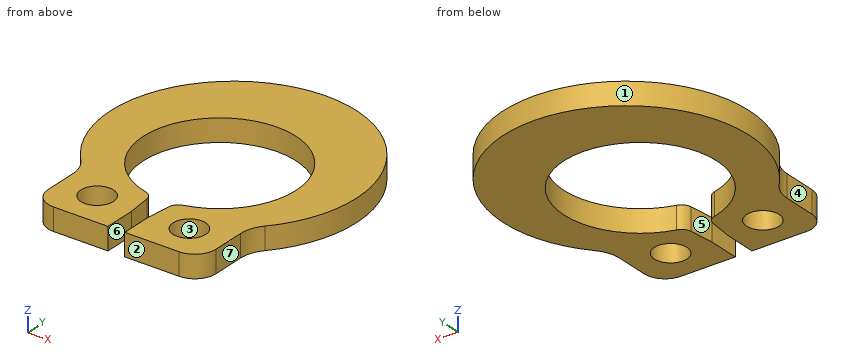
from build123d import *

# Parameters (mm, degrees)
SKETCH3_R               = 0.6477
BOSS_EXTRUDE1_DEPTH     = 0.4445
CUT_EXTRUDE1_DEPTH      = 1.4445
CUT_EXTRUDE1_DEPTH_BACK = 1.4445
FILLET1_R               = 0.4162425


with BuildPart() as part:
    # Sketch3 → Boss-Extrude1 (new body, symmetric)
    with BuildSketch(Plane.XY):
        with BuildLine():
            Line((3.32486, -4.653915), (3.32486, -3.346426518))
            ThreePointArc((3.32486, -3.346426518), (3.408862886, -2.887538523), (3.649976862, -2.488165606))
            ThreePointArc((3.649976862, -2.488165606), (0, 5.6134), (-3.649976862, -2.488165606))
            ThreePointArc((-3.649976862, -2.488165606), (-3.408862886, -2.887538523), (-3.32486, -3.346426518))
            Line((-3.32486, -3.346426518), (-3.32486, -4.653915))
            ThreePointArc((-3.32486, -4.653915), (-3.081030789, -5.242570789), (-2.492375, -5.4864))
            Line((-2.492375, -5.4864), (-0.332486, -5.4864))
            Line((-0.332486, -5.4864), (-0.332486, -3.004257615))
            ThreePointArc((-0.332486, -3.004257615), (0, 3.0226), (0.332486, -3.004257615))
            Line((0.332486, -3.004257615), (0.332486, -5.4864))
            Line((0.332486, -5.4864), (2.492375, -5.4864))
            ThreePointArc((2.492375, -5.4864), (3.081030789, -5.242570789), (3.32486, -4.653915))
        make_face()
        with Locations((-1.828673, -4.057999533)):
            Circle(SKETCH3_R, mode=Mode.SUBTRACT)
        with Locations((1.828673, -4.057999533)):
            Circle(SKETCH3_R, mode=Mode.SUBTRACT)
    extrude(amount=BOSS_EXTRUDE1_DEPTH, both=True)

    # Sketch4 → Cut-Extrude1 (cut, two sides)
    with BuildSketch(Plane.XY) as cut_extrude1_sk:
        Polygon((-0.332486, -4.245328808), (-0.797425121, 0), (0.797425121, 0), (0.332486, -4.245328808), align=None)
    extrude(amount=CUT_EXTRUDE1_DEPTH, mode=Mode.SUBTRACT)
    extrude(cut_extrude1_sk.sketch, amount=-CUT_EXTRUDE1_DEPTH_BACK, mode=Mode.SUBTRACT)

    # Fillet1
    fillet1_edges = [part.edges().sort_by_distance(p)[0] for p in [
        (-0.470430427, -2.985767234, 0),
        (0.470430427, -2.985767234, 0),
    ]]
    fillet(fillet1_edges, radius=FILLET1_R)


solid = part.part
For this review, take the finished solid that the model builds, in its own axes (mm). Face numbers are marked on the shaded views. A direction names the side the tool comes from. Give positions to 0.01 mm unless a question says otherwise; leave off trailing zeros. Loops run counter-clockwise (first coordinate to the right, second up) from the corner with the lowest first, then second, coordinate; pieces in that order, holes last. Notation, with made-up numbers: M 73.25,-25.75 L 130.25,-25.75 A19 cw 130.25,4.25 Z; hole C -30,-39 d6. An arc over 180 degrees is marked long. Put each result on its own line as item: value. Start each with the question number.
(1) For pin 1 (1.7 mm diameter, centred on x = 1.83, y = -4.06, fed in from +Z), flat-tipped, find the tip position at first contact; note if it passes through.
(2) The part is to be moulded in two halves that separate along Y. For the marked faces 1, 2 and 3, say which applies: +Y half, -Y half, draft (parallel to the pull), parting line (faces both ways), or undercut.
(3) Machinability: for the marked faces 4, 5, 6 and 7, which of the approach directions +Z, -Z, +X, -X, +Y, -Y give a long, thin tool a straight path to every point of the face, cutting with its end or side? Answer none if there is none.
(4) Wall thickness on L1, parallel to Y at x = 1.5, z = -0.15; L2, parallel to Y at x = 2, z = -0.4; L3, parallel to X at y = -4, z = 0.15: over which ranges is each line inside the solid? List them lowest first.
(5) Add section C-C, the plane z = 0. Write out the cut boundary in (x, y), then the cut area to 3 significant figures.
(6) Add section B-B, the plane y = 0. Write out the cut boundary in (x, z), then the cut area to 3 significant figures.
(7) Add section D-D, the plane x = 1.5. Write out the cut boundary in (y, z), then the cut area to 3 significant figures.
(8) Add section A-A, the plane x = -2.75. Write out the cut boundary in (y, z).
Result:
1. pin 1: stops at z = 0.44
2. face 1: parting line
2. face 2: -Y half
2. face 3: undercut
3. face 4: +Z, -Z, -X, -Y
3. face 5: +Z, -Z
3. face 6: +Z, -Z, -Y
3. face 7: +Z, -Z, +X, -Y
4. L1: y = -5.49 to -4.62, -3.5 to -2.62, 2.62 to 5.38
4. L2: y = -5.49 to -4.68, -3.43 to -2.27, 2.27 to 5.18
4. L3: x = -3.32 to -2.47, -1.18 to -0.36, 0.36 to 1.18, 2.47 to 3.32
5. outline: M -3.65,-2.49 A1.3 cw -3.32,-3.35 L -3.32,-4.65 A0.83 ccw -2.49,-5.49 L -0.33,-5.49 L -0.33,-4.25 L -0.44,-3.29 A0.42 ccw -0.75,-2.93 A3.02 cw long 0.75,-2.93 A0.42 ccw 0.44,-3.29 L 0.33,-4.25 L 0.33,-5.49 L 2.49,-5.49 A0.83 ccw 3.32,-4.65 L 3.32,-3.35 A1.3 cw 3.65,-2.49 A4.87 ccw long Z; hole C -1.83,-4.06 d1.3; hole C 1.83,-4.06 d1.3
5. area: 52.9 mm^2
6. outline: M -4.82,-0.44 L -3.02,-0.44 L -3.02,0.44 L -4.82,0.44 Z; M 3.02,-0.44 L 4.82,-0.44 L 4.82,0.44 L 3.02,0.44 Z
6. area: 3.19 mm^2
7. outline: M -5.49,-0.44 L -4.62,-0.44 L -4.62,0.44 L -5.49,0.44 Z; M -3.5,-0.44 L -2.62,-0.44 L -2.62,0.44 L -3.5,0.44 Z; M 2.62,-0.44 L 5.38,-0.44 L 5.38,0.44 L 2.62,0.44 Z
7. area: 4.00 mm^2
8. outline: M -5.45,-0.44 L -1.25,-0.44 L -1.25,0.44 L -5.45,0.44 Z; M 1.25,-0.44 L 4.76,-0.44 L 4.76,0.44 L 1.25,0.44 Z
